```python
from build123d import *

# Parameters (mm, degrees)
F0_W      = 102
F0_H      = 84
F0_R      = 2.25
F0_W_2    = 78
F0_H_2    = 51
F1_DEPTH  = 15
F3_DEPTH  = 4
F4_W      = 12
F4_H      = 44
F4_W_2    = 60
F4_H_2    = 13
F5_DEPTH  = 15.001
F6_W      = 102
F6_H      = 84
F7_DEPTH  = 8
F8_W      = 102
F8_H      = 25
F8_R      = 2.125
F9_DEPTH  = 10
F10_R     = 3.5
F11_DEPTH = 5
F12_R     = 5
F13_W     = 102
F13_H     = 5
F14_DEPTH = 15
F15_R     = 2.125
F16_DEPTH = 25
F17_R     = 7.5


with BuildPart() as f1:
    # F0 (on Top) → F1 (new body)
    with BuildSketch(Plane.XY):
        with Locations((0, -1.5)):
            Rectangle(F0_W, F0_H)
        with Locations((-44, -32.5)):
            Circle(F0_R, mode=Mode.SUBTRACT)
        with Locations((44, -32.5)):
            Circle(F0_R, mode=Mode.SUBTRACT)
        with Locations((-44, 32.5)):
            Circle(F0_R, mode=Mode.SUBTRACT)
        Rectangle(F0_W_2, F0_H_2, mode=Mode.SUBTRACT)
        with Locations((44, 32.5)):
            Circle(F0_R, mode=Mode.SUBTRACT)
    extrude(amount=F1_DEPTH)

    # F2 (on face) → F3 (cut)
    with BuildSketch(Plane(origin=(0, 0, 0), x_dir=(1, 0, 0), z_dir=(0, 0, -1))):
        Polygon((-41.075, 30.8112504626), (-41.075, 34.1887495374), (-44, 35.8774990748), (-46.925, 34.1887495374), (-46.925, 30.8112504626), (-44, 29.1225009252), align=None)
        Polygon((41.075, 34.1887495374), (41.075, 30.8112504626), (44, 29.1225009252), (46.925, 30.8112504626), (46.925, 34.1887495374), (44, 35.8774990748), align=None)
        Polygon((41.075, -30.8112504626), (41.075, -34.1887495374), (44, -35.8774990748), (46.925, -34.1887495374), (46.925, -30.8112504626), (44, -29.1225009252), align=None)
        Polygon((-41.075, -34.1887495374), (-41.075, -30.8112504626), (-44, -29.1225009252), (-46.925, -30.8112504626), (-46.925, -34.1887495374), (-44, -35.8774990748), align=None)
    extrude(amount=-F3_DEPTH, mode=Mode.SUBTRACT)

    # F4 (on face) → F5 (cut, through all)
    with BuildSketch(Plane.XY.offset(15)):
        with Locations((45, 3.5)):
            Rectangle(F4_W, F4_H)
        with Locations((1, -32)):
            Rectangle(F4_W_2, F4_H_2)
    extrude(amount=-F5_DEPTH, mode=Mode.SUBTRACT)

    # F6 (on face) → F7 (cut)
    with BuildSketch(Plane.XY.offset(15)):
        with Locations((0, -1.5)):
            Rectangle(F6_W, F6_H)
    extrude(amount=-F7_DEPTH, mode=Mode.SUBTRACT)

    # F8 (on face) → F9 (join)
    with BuildSketch(Plane.XY.offset(7)):
        with Locations((0, 53)):
            Rectangle(F8_W, F8_H)
        with Locations((-36, 53)):
            Circle(F8_R, mode=Mode.SUBTRACT)
        with Locations((0, 53)):
            Circle(F8_R, mode=Mode.SUBTRACT)
        with Locations((36, 53)):
            Circle(F8_R, mode=Mode.SUBTRACT)
    extrude(amount=-F9_DEPTH)

    # F10 (on face) → F11 (cut)
    with BuildSketch(Plane.XY.offset(7)):
        with Locations((36, 53)):
            Circle(F10_R)
        with Locations((0, 53)):
            Circle(F10_R)
        with Locations((-36, 53)):
            Circle(F10_R)
    extrude(amount=-F11_DEPTH, mode=Mode.SUBTRACT)

    # F12
    f12_edges = [f1.edges().sort_by_distance(p)[0] for p in [
        (-51, -43.5, 3.5),
        (51, -43.5, 3.5),
        (51, 25.5, 3.5),
        (51, -18.5, 3.5),
        (39, -18.5, 3.5),
        (31, -25.5, 3.5),
        (-29, -25.5, 3.5),
        (-51, 65.5, 2),
        (51, 65.5, 2),
    ]]
    fillet(f12_edges, radius=F12_R)

    # F13 (on face) → F14 (join)
    with BuildSketch(Plane(origin=(0, 0, -3), x_dir=(1, 0, 0), z_dir=(0, 0, -1))):
        with Locations((0, -43)):
            Rectangle(F13_W, F13_H)
    extrude(amount=F14_DEPTH)

    # F15 (on face) → F16 (cut)
    with BuildSketch(Plane.XZ.offset(-40.5)):
        with Locations((-31, -10.5)):
            Circle(F15_R)
        with Locations((31, -10.5)):
            Circle(F15_R)
    extrude(amount=-F16_DEPTH, mode=Mode.SUBTRACT)

    # F17
    f17_edges = [f1.edges().sort_by_distance(p)[0] for p in [
        (-51, 43, -18),
        (51, 43, -18),
    ]]
    fillet(f17_edges, radius=F17_R)


solid = f1.part
```
Here's how the part is built. I have some questions about the finished solid (model axes, mm). A direction names the side the tool comes from. Coordinates: 2 decimals unless noted, no trailing zeros. Order: outer loops, then holes, each group sorted by start corner. A loop starts at its lowest first (then second) coordinate and runs counter-clockwise, first axis right, second up. Notation, with made-up numbers: (29.5, -24) - (78.5, -24) arc R16 cw to (78.5, 7) - close; hole circle Ø11 at (-35.75, 48). An arc over 180 degrees is marked (long way). One line per question, with ' | ' between items.
(1) Suppose I cut it at D-D on y = 32.5. List the corners of the cut face in (x, z) for me (3 decimals), and give its area (3 significant figures).
Report:
outline: (-51, 0) - (-46.925, 0) - (-46.925, 4) - (-46.25, 4) - (-46.25, 7) - (-51, 7) - close; (-41.75, 4) - (-41.075, 4) - (-41.075, 0) - (41.075, 0) - (41.075, 4) - (41.75, 4) - (41.75, 7) - (-41.75, 7) - close; (46.25, 4) - (46.925, 4) - (46.925, 0) - (51, 0) - (51, 7) - (46.25, 7) - close | area: 640 mm2
(2) Suppose I cut it at A-A on x = 15. List the corners of the cut face in (y, z) for me.
Report:
outline: (-43.5, 0) - (-38.5, 0) - (-38.5, 7) - (-43.5, 7) - close; (25.5, 0) - (40.5, 0) - (40.5, -18) - (45.5, -18) - (45.5, -3) - (65.5, -3) - (65.5, 7) - (25.5, 7) - close
(3) Suppose I cut it at B-B on y = -32.5. List the corners of the cut face in (x, z) for me (3 decimals), and give its area (3 significant figures).
Report:
outline: (-51, 0) - (-46.925, 0) - (-46.925, 4) - (-46.25, 4) - (-46.25, 7) - (-51, 7) - close; (-41.75, 4) - (-41.075, 4) - (-41.075, 0) - (-29, 0) - (-29, 7) - (-41.75, 7) - close; (31, 0) - (41.075, 0) - (41.075, 4) - (41.75, 4) - (41.75, 7) - (31, 7) - close; (46.25, 4) - (46.925, 4) - (46.925, 0) - (51, 0) - (51, 7) - (46.25, 7) - close | area: 220 mm2
(4) Will these pins go through, and if not, where does the flat tip stop? pin 1 (5.5 mm diameter, centred on x = -18, z = -8, fed in from -Y); pin 2 (8 mm diameter, centred on x = 36, y = 53, fed in from -Z); pin 3 (6.5 mm diameter, centred on x = -36, y = 53, fed in from +Z).
Report:
pin 1: stops at y = 40.5 | pin 2: stops at z = -3 | pin 3: stops at z = 2
(5) If we mould it in two halves opening along Y, with no side actions, what happens to faces 1 (the cylindrical face through (49.5, -42.07, 3.55)), 2 (the flat face through (-45.483, 35.021, 1.972)), 3 (the flat face through (-51, 12, 2))? For each: pulls with the +Y half, pulls with the -Y half, needs draft (parallel to the pull), parting line crosses it, or undercut.
Report:
face 1: pulls with the -Y half | face 2: undercut | face 3: needs draft
(6) For faces 4 (the flat face through (41.075, -33, 2)), 5 (the cylindrical face through (-30.5, -26.93, 3.45)), 6 (the cylindrical face through (33.42, 55.365, 4.535)), which set-ups out of +Z, -Z, +X, -X, +Y, -Y let a thin tool reach every point of the face, with its end or its side?
Report:
face 4: -Z | face 5: +Z, -Z | face 6: +Z
(7) If I drill on L1, parallel to Y at x = 0, z = 5.05; L2, parallel to Y at x = -44, z = 5.5; L3, parallel to Z at x = 31, y = 41.7 (3 decimals), over which ranges is the centre line in solid material (lowest first)?
Report:
L1: y = -43.5 to -38.5, 25.5 to 49.5, 56.5 to 65.5 | L2: y = -43.5 to -34.75, -30.25 to 30.25, 34.75 to 65.5 | L3: z = -18 to -12.625, -8.375 to 7
(8) Suppose I cut it at C-C on x = 0. List the corners of the cut face in (y, z) for me (3 decimals).
Report:
outline: (-43.5, 0) - (-38.5, 0) - (-38.5, 7) - (-43.5, 7) - close; (25.5, 0) - (40.5, 0) - (40.5, -18) - (45.5, -18) - (45.5, -3) - (50.875, -3) - (50.875, 2) - (49.5, 2) - (49.5, 7) - (25.5, 7) - close; (55.125, -3) - (65.5, -3) - (65.5, 7) - (56.5, 7) - (56.5, 2) - (55.125, 2) - close
